```python
from build123d import *

# Parameters (mm, degrees)
F1_W     = 203.2
F1_H     = 101.6
F2_DEPTH = 5.08
F5_DEPTH = 25.4


with BuildPart() as f2:
    # F1 (on Front) → F2 (new body)
    with BuildSketch(Plane.XZ):
        with Locations((101.6, 50.8)):
            Rectangle(F1_W, F1_H)
    extrude(amount=-F2_DEPTH)

    # F4 (on face) → F5 (cut)
    with BuildSketch(Plane.XZ):
        Polygon((19.05, 88.9), (6.35, 63.4896950778), (6.35, 54.3535576701), (19.05, 79.7638625923), align=None)
        Polygon((19.05, 44.7899766155), (6.35, 38.9748217106), (6.35, 26.9433392146), (19.05, 20.5959144004), (19.05, 31.75), align=None)
        Polygon((25.4, 64.1602875233), (25.4, 50.8), (25.3980111729, 41.5485496718), (38.1, 31.75), (38.1, 50.8), (38.1, 64.1602875233), align=None)
        Polygon((25.4, 88.9), (25.4, 64.1602875233), (38.1, 64.1602875233), (38.1, 64.2026114812), align=None)
        Polygon((57.15, 88.9), (44.45, 88.9), (44.45, 63.2637151304), (48.3517487947, 51.1962487751), (44.45, 31.964471331), (50.8, 12.7), (57.15, 31.964471331), (53.2482512053, 51.1962487751), (50.8, 63.2637151304), align=None)
        Polygon((76.2, 76.2), (63.5, 88.9), (63.5, 38.0811007293), (76.2, 44.45), (78.4824932634, 32.6018280187), (90.3535660462, 38.1168511729), (87.9102185152, 50.8), (91.5801092576, 57.15), (76.2, 57.15), align=None)
        Polygon((76.2, 37.8645947099), (63.5, 31.964471331), (63.5, 25.7733563287), (76.2, 25.7733563287), align=None)
        Polygon((133.35, 50.8), (114.3, 57.15), (101.6, 50.8), (114.3, 44.45), align=None)
        Polygon((114.3, 44.45), (101.6, 50.8), (101.6, 30.8501303583), (114.3, 36.4221383274), align=None)
        Polygon((108.9507660084, 88.9), (114.3, 76.2), (133.35, 76.2), (133.35, 88.9), align=None)
        Polygon((133.35, 25.4), (114.3, 25.4), (127.2270479083, 12.7), (133.35, 12.7643318847), align=None)
        Polygon((149.225, 76.2), (152.4, 76.2), (158.75, 88.9), (139.7, 88.9), (139.7, 53.975), align=None)
        Polygon((158.75, 88.9), (152.4, 76.2), (155.575, 63.5), (161.925, 63.5), (165.1, 76.2), align=None)
        Polygon((177.8, 53.975), (177.8, 88.9), (168.275, 76.2), (168.275, 65.0875), align=None)
        Polygon((177.8, 47.625), (139.7, 47.625), (139.7, 26.9875), (149.225, 36.5125), (149.225, 38.1), (171.658446914, 38.1), align=None)
        Polygon((149.225, 23.8125), (139.7, 23.8125), (139.7, 12.7), (150.6915916045, 12.7), (150.6915916045, 22.225), (149.225, 22.225), align=None)
        Polygon((196.85, 88.9), (189.7574476064, 38.1), (193.675, 38.1), align=None)
        Polygon((196.85, 12.7), (189.7574476064, 29.845), (187.325, 29.845), (184.3011081219, 12.7), align=None)
    extrude(amount=-F5_DEPTH, mode=Mode.SUBTRACT)


solid = f2.part
```
Can you work these out from the model? Positions are in its coordinate system, mm. Round coordinates to 2 decimals unless told otherwise and drop trailing zeros. Loops run counter-clockwise (first coordinate to the right, second up) from the corner with the lowest first, then second, coordinate; pieces in that order, holes last.
Item 1: Please list where these lines run through material, in increasing order: L1, parallel to Z at x = 157, y = 2.1 (3 decimals); L2, parallel to Z at x = 14.5, y = 1.6; L3, parallel to X at y = 0.95, z = 22.
Item 2: Will this pin go through, and if not, where does the flat tip stop? pin 1 Ø1 at (x, z) = (46.5, 37.5) entering from +Y.
Item 3: Suppose I cut it at B-B, the plane z = 69. State how many separate pieces and enclosed holes the cut face has, then the cut area to 3 significant figures.
Item 4: If we mould it in two halves opening along X, with no side actions, what happens to faces 1 (the flat face through (100, 5.08, 52)), 2 (the flat face through (177.8, 3, 71))? For each: +X half, -X half, draft (parallel to the pull), parting line (faces both ways), or undercut.
Item 5: Suppose I cut it at A-A, the plane x = 33. Write out the boundary of the cut face in (y, z), then the cut area to 3 significant figures.
Reported:
1. L1: z = 0 to 38.1, 47.625 to 63.5, 88.9 to 101.6
1. L2: z = 0 to 22.87, 42.71 to 70.66, 79.8 to 101.6
1. L3: x = 0 to 16.24, 19.05 to 47.73, 53.87 to 117.76, 133.35 to 139.7, 150.69 to 185.94, 193 to 203.2
2. pin 1: passes through
3. separate pieces: 9
3. enclosed holes: 0
3. area: 718 mm2
4. face 1: draft
4. face 2: undercut
5. outline: (0, 0) - (5.08, 0) - (5.08, 35.68) - (0, 35.68) - close; (0, 74.12) - (5.08, 74.12) - (5.08, 101.6) - (0, 101.6) - close
5. area: 321 mm2
